from build123d import *

# Parameters (mm, degrees)
SKETCH1_R                = 7.5
BOSS_EXTRUDE1_DEPTH      = 100
SKETCH2_W                = 5
SKETCH2_H                = 45
BOSS_EXTRUDE3_DEPTH      = 9.5
CUT_EXTRUDE1_START       = -10
CUT_EXTRUDE1_DEPTH       = 10
FILLET1_R                = 1
CIRPATTERN8_COUNT        = 7
FILLET1_OF_CIRPATTERN8_R = 1
FILLET3_R                = 0.25


with BuildPart() as part:
    # Sketch1 → Boss-Extrude1 (new body)
    with BuildSketch(Plane.XY):
        Circle(SKETCH1_R)
    extrude(amount=BOSS_EXTRUDE1_DEPTH)

    # Sketch2 → Boss-Extrude3 (add)
    with BuildSketch(Plane(origin=(0, 0, 0), x_dir=(1, 0, 0), z_dir=(0, 1, 0))):
        with Locations((0, -28.25)):
            Rectangle(SKETCH2_W, SKETCH2_H)
    extrude(amount=BOSS_EXTRUDE3_DEPTH)

    # Sketch3 → Cut-Extrude1 (cut)
    with BuildSketch(Plane.XY.offset(100).offset(CUT_EXTRUDE1_START)):
        with BuildLine():
            ThreePointArc((2.5, 7.071067812), (0, 7.5), (-2.5, 7.071067812))
            Line((-2.5, 7.071067812), (-2.166666667, 6.12825877))
            ThreePointArc((-2.166666667, 6.12825877), (0, 6.5), (2.166666667, 6.12825877))
            Line((2.166666667, 6.12825877), (2.5, 7.071067812))
        make_face()
    cut_extrude1 = extrude(amount=CUT_EXTRUDE1_DEPTH, mode=Mode.SUBTRACT)

    # Fillet1
    # the kernel refuses this fillet: 1 mm, written as the material it takes off along each edge
    with BuildSketch(Plane(origin=(2.5, 7.071067812, 90), x_dir=(0.9143745015294013, -0.4048694492708226, 0), z_dir=(0, 0, 1))) as fillet1_piece_1:
        with BuildLine():
            CenterArc((1.076923077, -0.997037031), FILLET1_R, 85.588274214, 94.411725786)
            Line((0.076923077, -0.997037031), (0.056923077, -0.997037031))
            ThreePointArc((0.056923077, -0.997037031), (0.018520798, -0.500056977), (-0.019940741, -0.001538462))
            Line((-0.019940741, -0.001538462), (-0.001538462, 0.019940741))
            ThreePointArc((-0.001538462, 0.019940741), (0.576923077, 0.042222271), (1.155384615, 0.019940741))
            Line((1.155384615, 0.019940741), (1.153846154, 0))
        make_face()
    extrude(amount=12.884615385, mode=Mode.SUBTRACT)
    with BuildSketch(Plane(origin=(-2.5, 7.071067812, 90), x_dir=(-0.9143745015294016, -0.40486944927082136, 0), z_dir=(0, 0, 1))) as fillet1_piece_2:
        with BuildLine():
            CenterArc((1.076923077, 0.997037031), FILLET1_R, 180, 94.411725786)
            Line((0.076923077, 0.997037031), (0.056923077, 0.997037031))
            ThreePointArc((0.056923077, 0.997037031), (0.018520798, 0.500056977), (-0.019940741, 0.001538462))
            Line((-0.019940741, 0.001538462), (-0.001538462, -0.019940741))
            ThreePointArc((-0.001538462, -0.019940741), (0.576923077, -0.042222271), (1.155384615, -0.019940741))
            Line((1.155384615, -0.019940741), (1.153846154, 0))
        make_face()
    extrude(amount=12.884615385, mode=Mode.SUBTRACT)

    # CirPattern8: Cut-Extrude1 ×7 about axis
    cirpattern8_axis = Axis((0, 0, 0), (0, 0, 1))
    for i in range(1, CIRPATTERN8_COUNT):
        add(cut_extrude1.rotate(cirpattern8_axis, i * 360 / CIRPATTERN8_COUNT), mode=Mode.SUBTRACT)

    # Fillet1 of CirPattern8
    # the kernel refuses this fillet: 1 mm, written as the material it takes off along each edge
    with BuildSketch(Plane(origin=(-3.969658925, 6.363317375, 90), x_dir=(0.8866428585126668, 0.4624547993571771, 0), z_dir=(0, 0, 1)), Plane(origin=(-7.450083714, 0.863859167, 90), x_dir=(0.19125105881764654, 0.9815411517104767, 0), z_dir=(0, 0, 1)), Plane(origin=(-5.320443512, -5.286102614, 90), x_dir=(-0.6481566889776921, 0.7615069970351391, 0), z_dir=(0, 0, 1)), Plane(origin=(0.815599172, -7.455521309, 90), x_dir=(-0.9994892299858744, -0.031957458319521785, 0), z_dir=(0, 0, 1)), Plane(origin=(6.337479044, -4.010780394, 90), x_dir=(-0.5981859949499692, -0.8013572957462329, 0), z_dir=(0, 0, 1)), Plane(origin=(7.087107935, 2.454159963, 90), x_dir=(0.25356349505382336, -0.9673187447662169, 0), z_dir=(0, 0, 1))) as fillet1_of_cirpattern8_piece_1:
        with BuildLine():
            CenterArc((1.076923077, -0.997037031), FILLET1_OF_CIRPATTERN8_R, 85.588274214, 94.411725786)
            Line((0.076923077, -0.997037031), (0.056923077, -0.997037031))
            ThreePointArc((0.056923077, -0.997037031), (0.018520798, -0.500056977), (-0.019940741, -0.001538462))
            Line((-0.019940741, -0.001538462), (-0.001538462, 0.019940741))
            ThreePointArc((-0.001538462, 0.019940741), (0.576923077, 0.042222271), (1.155384615, 0.019940741))
            Line((1.155384615, 0.019940741), (1.153846154, 0))
        make_face()
    extrude(amount=12.884615385, mode=Mode.SUBTRACT)
    with BuildSketch(Plane(origin=(-7.087107935, 2.454159963, 90), x_dir=(-0.25356349505382375, -0.9673187447662169, 0), z_dir=(0, 0, 1)), Plane(origin=(-6.337479044, -4.010780394, 90), x_dir=(0.5981859949499683, -0.8013572957462336, 0), z_dir=(0, 0, 1)), Plane(origin=(-0.815599172, -7.455521309, 90), x_dir=(0.9994892299858742, -0.03195745831952264, 0), z_dir=(0, 0, 1)), Plane(origin=(5.320443512, -5.286102614, 90), x_dir=(0.6481566889776939, 0.7615069970351375, 0), z_dir=(0, 0, 1)), Plane(origin=(7.450083714, 0.863859167, 90), x_dir=(-0.1912510588176455, 0.981541151710477, 0), z_dir=(0, 0, 1)), Plane(origin=(3.969658925, 6.363317375, 90), x_dir=(-0.8866428585126658, 0.46245479935717904, 0), z_dir=(0, 0, 1))) as fillet1_of_cirpattern8_piece_2:
        with BuildLine():
            CenterArc((1.076923077, 0.997037031), FILLET1_OF_CIRPATTERN8_R, 180, 94.411725786)
            Line((0.076923077, 0.997037031), (0.056923077, 0.997037031))
            ThreePointArc((0.056923077, 0.997037031), (0.018520798, 0.500056977), (-0.019940741, 0.001538462))
            Line((-0.019940741, 0.001538462), (-0.001538462, -0.019940741))
            ThreePointArc((-0.001538462, -0.019940741), (0.576923077, -0.042222271), (1.155384615, -0.019940741))
            Line((1.155384615, -0.019940741), (1.153846154, 0))
        make_face()
    extrude(amount=12.884615385, mode=Mode.SUBTRACT)

    # Fillet3
    fillet3_edges = [part.edges().sort_by_distance(p)[0] for p in [
        (0, 9.5, 50.75),
        (-2.5, 9.5, 28.25),
        (-7.5, 0, 0),
        (-2.5, 7.071067812, 28.25),
        (0, 7.5, 5.75),
        (2.5, 7.071067812, 28.25),
        (0, 7.5, 50.75),
        (2.5, 9.5, 28.25),
        (2.5, 8.285533906, 50.75),
        (-2.5, 8.285533906, 5.75),
        (-2.5, 8.285533906, 50.75),
        (0, 9.5, 5.75),
        (2.5, 8.285533906, 5.75),
    ]]
    fillet(fillet3_edges, radius=FILLET3_R)


solid = part.part
Can you work these out from the model? Positions are in its coordinate system, mm. A direction names the side the tool comes from. Round coordinates to 2 decimals unless told otherwise and drop trailing zeros. Order: outer loops, then holes, each group sorted by start corner. A loop starts at its lowest first (then second) coordinate and runs counter-clockwise, first axis right, second up. Notation, with made-up numbers: (18.25, -28.5) -> (31.25, -28.5) arc R21 cw to (31.25, 4.5) -> close; hole circle Ø8 at (74, -4.5). An arc over 180 degrees is marked (long way). Write each question's results on one line, items separated by ' | '. Start each with the question number.
Item 1: If we section it at B-B, the plane z = 88.5: Write out the boundary of the cut face in (x, y), then the cut area to 3 significant figures.
Item 2: Thinking about a two-plate mould opening in Y: for faces 1 (the flat face through (0, 9, 50.75)), 2 (the cylindrical face through (6.344, -1.416, 94.93)), 3 (the cylindrical face through (3.461, -6.654, 44.497)), which applies, +Y half, -Y half, draft (parallel to the pull), parting line (faces both ways), or undercut?
Item 3: Which directions (+Z, -Z, +X, -X, +Y, -Y) give clear straight access to the entire face, cutting with the end or side of a thin tool? Please do faces 4 (the flat face through (-6, 3, 90)), 5 (the cylindrical face through (0, 6.5, 94.9)), 6 (the flat face through (2.5, 8, 29)), 7 (the flat face through (-2.5, 8, 29)).
Item 4: Please list where these lines run through material, in increasing order: L1, parallel to X at y = 7.75, z = 41.5; L2, parallel to X at y = -1, z = 67; L3, parallel to Z at x = -3.5, y = -6.
Item 5: Will these pins go through, and if not, where does the flat tip stop? pin 1 (0.9 mm diameter, centred on x = 0.5, y = 8.5, fed in from -Z); pin 2 (6 mm diameter, centred on y = 7.5, z = 64.5, fed in from +X); pin 3 (1.6 mm diameter, centred on y = 8, z = 32, fed in from -X).
Item 6: If we section it at A-A, the plane z = 19: Write out the boundary of the cut face in (x, y).
Results:
1) outline: circle Ø15 at (0, 0) | area: 177 mm2
2) face 1: draft | face 2: undercut | face 3: parting line
3) face 4: +Z | face 5: +Z, +Y | face 6: +Z, -Z, +X, +Y | face 7: +Z, -Z, -X, +Y
4) L1: x = -2.5 to 2.5 | L2: x = -7.43 to 7.43 | L3: z = 0 to 90
5) pin 1: stops at z = 5.75 | pin 2: stops at x = 6 | pin 3: stops at x = -2.5
6) outline: (-2.66, 7.01) arc R7.5 ccw (long way) to (2.66, 7.01) arc R0.25 cw to (2.5, 7.25) -> (2.5, 9.25) arc R0.25 ccw to (2.25, 9.5) -> (-2.25, 9.5) arc R0.25 ccw to (-2.5, 9.25) -> (-2.5, 7.25) arc R0.25 cw to start
